Verification items for the finished model (mm, model axes). Give positions to 0.01 mm unless a question says otherwise; leave off trailing zeros. Order: outer loops, then holes, each group sorted by start corner. A loop starts at its lowest first (then second) coordinate and runs counter-clockwise, first axis right, second up.
from build123d import *

# Parameters (mm, degrees)
SHELL1_T            = 2
SKETCH2_R           = 125.720178412
CUT_EXTRUDE1_DEPTH  = 156
SKETCH3_R           = 99
SKETCH3_R_2         = 98
BOSS_EXTRUDE1_DEPTH = 3.8


with BuildPart() as part:
    # Sketch1 → Revolve1 (revolve)
    with BuildSketch(Plane(origin=(0, 0, 0), x_dir=(1, 0, 0), z_dir=(0, 1, 0))):
        with BuildLine():
            Line((0, 100), (0, -100))
            ThreePointArc((0, -100), (100, 0), (0, 100))
        make_face()
    revolve(axis=Axis((0, 0, -100), (0, 0, 1)))

    # Shell1 (no face opened: a closed hollow body)
    add(offset(amount=-SHELL1_T, mode=Mode.PRIVATE), mode=Mode.SUBTRACT)

    # Sketch2 → Cut-Extrude1 (cut)
    with BuildSketch(Plane(origin=(0, 0, 0), x_dir=(1, 0, 0), z_dir=(0, 1, 0))):
        Circle(SKETCH2_R)
    extrude(amount=CUT_EXTRUDE1_DEPTH, mode=Mode.SUBTRACT)

    # Sketch3 → Boss-Extrude1 (add)
    with BuildSketch(Plane(origin=(0, 0, 0), x_dir=(1, 0, 0), z_dir=(0, 1, 0))):
        with Locations(Location((0, 0, 0), (0, 0, 90))):
            Circle(SKETCH3_R)
        with Locations(Location((0, 0, 0), (0, 0, 90))):
            Circle(SKETCH3_R_2, mode=Mode.SUBTRACT)
    extrude(amount=BOSS_EXTRUDE1_DEPTH)


solid = part.part
(1) Section check C-C, the plane y = -45.5. Enter the section's corners in (x, z), then the cut area to 3 significant figures.
Solved:
outline: circle Ø178.1 at (0, 0); hole circle Ø173.59 at (0, 0)
area: 1,240 mm2
(2) Section check A-A, the plane x = 0. Enter the section's corners in (y, z), then the cut area to 3 significant figures.
Solved:
outline: (0, -100) - (0, -99) - (3.8, -99) - (3.8, -98) - (0, -98) arc R98 cw to (0, 98) - (3.8, 98) - (3.8, 99) - (0, 99) - (0, 100) arc R100 ccw to start
area: 630 mm2
(3) Scan lines: line 1 (X direction, y = 2.95, z = 0); line 2 (X direction, y = -74.5, z = -7); line 3 (Z direction, x = -35, y = -65.5). Record each from-to range of solid material in increasing order.
Solved:
line 1: x = -99 to -98, 98 to 99
line 2: x = -66.34 to -63.28, 63.28 to 66.34
line 3: z = -66.97 to -63.94, 63.94 to 66.97
(4) Go/stop test with flat-tipped pins: pin 1 (8 mm diameter, centred on y = -52.5, z = -32, fed in from +X); pin 2 (1 mm diameter, centred on x = -14, y = -72.5, fed in from -Z); pin 3 (4 mm diameter, centred on x = -29, z = 20, fed in from -Y). Record where each tip stops, or that it passes through.
Solved:
pin 1: stops at x = 81.83
pin 2: stops at z = -67.98
pin 3: stops at y = -94.32
(5) Release check for a two-part mould opening along Z. For faces 1 (the cylindrical face through (-66.909, 1.873, 72.967)), 2 (the flat face through (-97, 0, -23)), 3 (the cylindrical face through (-29.437, 1.873, -93.475)) record: pulls with the +Z half, pulls with the -Z half, needs draft (parallel to the pull), parting line crosses it, or undercut.
Solved:
face 1: parting line crosses it
face 2: needs draft
face 3: undercut
(6) Section check B-B, the plane z = 0. Enter the section's corners in (x, y), then the cut area to 3 significant figures.
Solved:
outline: (-100, 0) arc R100 ccw to (100, 0) - (99, 0) - (99, 3.8) - (98, 3.8) - (98, 0) arc R98 cw to (-98, 0) - (-98, 3.8) - (-99, 3.8) - (-99, 0) - close
area: 630 mm2
